Input: part model. Units: mm. Frame: model coordinates. Round coordinates to 2 decimals unless told otherwise and drop trailing zeros. Loops run counter-clockwise (first coordinate to the right, second up) from the corner with the lowest first, then second, coordinate; pieces in that order, holes last. Notation, with made-up numbers: (34, 14.25) - (87, 14.25) arc R35 cw to (87, 50.25) - close; hole circle Ø5 at (79.5, 50). An arc over 180 degrees is marked (long way). One line per question, with ' | ' between items. Start each with the question number.
Item 1: Section C-C, the plane y = -98.5. Return loops of the section in (x, z).
Item 2: Section B-B, the plane y = -84.5. Return loops of the section in (x, z), plus the area to 3 significant figures.
Item 3: First-contact query: pin 1 (0.5 mm diameter, centred on x = -110.5, z = 0.5, fed in from -Y); pin 2 (0.5 mm diameter, centred on y = -97.5, z = 0.5, fed in from +X). Flat tips, straight axial feed; report the tip coordinate or a pass-through.
Item 4: Draft query along Y for faces 1 (the face through (-128.56, -108.89, 0.49)), 2 (the face through (-85, -63, 0.5)), 3 (the face through (-133.83, -111.824, 0.493)). Return one class per face: pulls with the +Y half, pulls with the -Y half, needs draft (parallel to the pull), parting line crosses it, or undercut.
Item 5: Section D-D, the plane z = 0.15. Give the number of separate pieces and of enclosed holes in the cut face, plus the area to 3 significant figures.
Item 6: Section A-A, the plane x = -114.5. Return loops of the section in (y, z).
Item 7: Material intervals for line 1 along Y through (x, z) = (-113, 0.65); line 2 along Y through (x, z) = (-106, 0.15); line 3 along X through (y, z) = (-96, 0.1), sorted ascending.
```python
from build123d import *

# Parameters (mm, degrees)
ESQUISSE1_R        = 1.745730463
ESQUISSE1_R_2      = 1.75
ESQUISSE1_W        = 8.004851144
ESQUISSE1_H        = 8.004851144
BOSS_EXTRU_1_DEPTH = 1


with BuildPart() as part:
    # Esquisse1 → Boss.-Extru.1 (new body)
    with BuildSketch(Plane.XY):
        with BuildLine():
            Line((-122.090539275, -67.2444), (-98.063455394, -67.2444))
            Line((-98.063455394, -67.2444), (-96.772260725, -67.2444))
            ThreePointArc((-96.772260725, -67.2444), (-96.065153944, -66.951506781), (-95.772260725, -66.2444))
            Line((-95.772260725, -66.2444), (-95.772260725, -63.394))
            ThreePointArc((-95.772260725, -63.394), (-95.479367507, -62.686893219), (-94.772260725, -62.394))
            Line((-94.772260725, -62.394), (-86.4314, -62.394))
            ThreePointArc((-86.4314, -62.394), (-85.017186438, -62.979786438), (-84.4314, -64.394))
            Line((-84.4314, -64.394), (-84.4314, -70.310741156))
            ThreePointArc((-84.4314, -70.310741156), (-84.724293219, -71.017847937), (-85.4314, -71.310741156))
            Line((-85.4314, -71.310741156), (-94.772260725, -71.310741156))
            ThreePointArc((-94.772260725, -71.310741156), (-95.479367507, -71.603634375), (-95.772260725, -72.310741156))
            Line((-95.772260725, -72.310741156), (-95.772260725, -106.5436))
            ThreePointArc((-95.772260725, -106.5436), (-96.065153944, -107.250706781), (-96.772260725, -107.5436))
            Line((-96.772260725, -107.5436), (-110.749678549, -107.5436))
            ThreePointArc((-110.749678549, -107.5436), (-111.45678533, -107.836493219), (-111.749678549, -108.5436))
            Line((-111.749678549, -108.5436), (-111.749678549, -111.394))
            ThreePointArc((-111.749678549, -111.394), (-112.042571768, -112.101106781), (-112.749678549, -112.394))
            Line((-112.749678549, -112.394), (-132.4314, -112.394))
            ThreePointArc((-132.4314, -112.394), (-133.845613562, -111.808213562), (-134.4314, -110.394))
            Line((-134.4314, -110.394), (-134.4314, -103.6932))
            ThreePointArc((-134.4314, -103.6932), (-134.138506781, -102.986093219), (-133.4314, -102.6932))
            Line((-133.4314, -102.6932), (-124.090539275, -102.6932))
            ThreePointArc((-124.090539275, -102.6932), (-123.383432493, -102.400306781), (-123.090539275, -101.6932))
            Line((-123.090539275, -101.6932), (-123.090539275, -68.2444))
            ThreePointArc((-123.090539275, -68.2444), (-122.797646056, -67.537293219), (-122.090539275, -67.2444))
        make_face()
        with Locations((-130.170361884, -108.219670908)):
            Circle(ESQUISSE1_R, mode=Mode.SUBTRACT)
        with Locations((-88.817, -66.847)):
            Circle(ESQUISSE1_R_2, mode=Mode.SUBTRACT)
        with Locations((-109.4314, -87.394)):
            Rectangle(ESQUISSE1_W, ESQUISSE1_H, mode=Mode.SUBTRACT)
        with BuildLine():
            Line((-118.004092872, -71.30163173), (-100.936518074, -71.30163173))
            ThreePointArc((-100.936518074, -71.30163173), (-100.229411293, -71.594524949), (-99.936518074, -72.30163173))
            Line((-99.936518074, -72.30163173), (-99.936518074, -79.429611883))
            ThreePointArc((-99.936518074, -79.429611883), (-100.229411293, -80.136718664), (-100.936518074, -80.429611883))
            Line((-100.936518074, -80.429611883), (-118.004092872, -80.429611883))
            ThreePointArc((-118.004092872, -80.429611883), (-118.711199653, -80.136718664), (-119.004092872, -79.429611883))
            Line((-119.004092872, -79.429611883), (-119.004092872, -72.30163173))
            ThreePointArc((-119.004092872, -72.30163173), (-118.711199653, -71.594524949), (-118.004092872, -71.30163173))
        make_face(mode=Mode.SUBTRACT)
        with BuildLine():
            Line((-118.004092872, -103.48636827), (-100.936518074, -103.48636827))
            ThreePointArc((-100.936518074, -103.48636827), (-100.229411293, -103.193475051), (-99.936518074, -102.48636827))
            Line((-99.936518074, -102.48636827), (-99.936518074, -95.358388117))
            ThreePointArc((-99.936518074, -95.358388117), (-100.229411293, -94.651281336), (-100.936518074, -94.358388117))
            Line((-100.936518074, -94.358388117), (-118.004092872, -94.358388117))
            ThreePointArc((-118.004092872, -94.358388117), (-118.711199653, -94.651281336), (-119.004092872, -95.358388117))
            Line((-119.004092872, -95.358388117), (-119.004092872, -102.48636827))
            ThreePointArc((-119.004092872, -102.48636827), (-118.711199653, -103.193475051), (-118.004092872, -103.48636827))
        make_face(mode=Mode.SUBTRACT)
    extrude(amount=BOSS_EXTRU_1_DEPTH)


solid = part.part
```
Return value:
1) outline: (-123.09, 0) - (-119, 0) - (-119, 1) - (-123.09, 1) - close; (-99.94, 0) - (-95.77, 0) - (-95.77, 1) - (-99.94, 1) - close
2) outline: (-123.09, 0) - (-113.43, 0) - (-113.43, 1) - (-123.09, 1) - close; (-105.43, 0) - (-95.77, 0) - (-95.77, 1) - (-105.43, 1) - close | area: 19.3 mm2
3) pin 1: y = -107.54 | pin 2: x = -95.77
4) face 1: undercut | face 2: pulls with the +Y half | face 3: pulls with the -Y half
5) separate pieces: 1 | enclosed holes: 5 | area: 935 mm2
6) outline: (-112.39, 0) - (-103.49, 0) - (-103.49, 1) - (-112.39, 1) - close; (-94.36, 0) - (-80.43, 0) - (-80.43, 1) - (-94.36, 1) - close; (-71.3, 0) - (-67.24, 0) - (-67.24, 1) - (-71.3, 1) - close
7) line 1: -112.39 to -103.49, -94.36 to -91.4, -83.39 to -80.43, -71.3 to -67.24 | line 2: -107.54 to -103.49, -94.36 to -91.4, -83.39 to -80.43, -71.3 to -67.24 | line 3: -123.09 to -119, -99.94 to -95.77
